Geometry: final body of the model. Coordinates: model frame, mm. A direction names the side the tool comes from. Coordinates: 2 decimals unless noted, no trailing zeros. Order: outer loops, then holes, each group sorted by start corner. A loop starts at its lowest first (then second) coordinate and runs counter-clockwise, first axis right, second up. Notation, with made-up numbers: M -8.5,65 L 3.5,65 A33 ccw 3.5,104 Z; hole C 74,6.5 d5. An arc over 180 degrees is marked long. Use CSV: the item, a comma, the result in double quotes. Start each with the question number.
Q1. Section query C-C, the plane y = 1.5. Output: boundary loops of the cut face in (x, z), and give its area (3 significant figures).
Q2. Mould query, pull axis Y, two halves, no side actions, for faces 1 (the face through (1, -1.828, -15)), 2 (the face through (-22.1, -4.1, -0.7)), 3 (the face through (22.4, -3.128, -6.2)), 4 (the face through (18, -13.128, 4)). Classes: +Y half, -Y half, draft (parallel to the pull), parting line (faces both ways), or undercut.
Q3. Section query B-B, the plane z = 30.5. Output: boundary loops of the cut face in (x, y), and give its area (3 significant figures).
Q4. Ray query, probe 1 along X at (y, z) = (-2.5, -1); probe 2 along Y at (x, z) = (-21, -10); probe 3 along Z at (x, y) = (11.5, -9.25). Return the intervals inside material, ascending.
Q5. First-contact query: P1, Ø1.5, axis at y = -11, z = 16.5, coming from the -X side; P2, Ø11.5, axis at x = -25.02, z = 0, coming from the -Y side; P3, Ø2, axis at x = -6.5, z = -4, coming from the +Y side; P4, Ø5.5, axis at x = 7.48, z = 32.5, coming from the -Y side. Flat tips, straight axial feed; report the tip coordinate or a pass-through.
Q6. Access query for faces 5 (the face through (-1, -17.128, -9)), 6 (the face through (3.51, -0.09, -29.46)), 7 (the face through (26, -5.128, -8)). Directions: +Z, -Z, +X, -X, +Y, -Y. A direction counts if a zero-diameter tool reaches every point of the face in a straight line with its end or side. Return the directions, or none.
Q7. Section query A-A, the plane z = 0. State how many separate pieces and enclosed holes the cut face has, and give its area (3 significant figures).
from build123d import *

# Parameters (mm, degrees)
F3_D            = 6
F3_COPIES_COUNT = 4
F4_R            = 5
F4_R_2          = 3
F5_DEPTH        = 6
F5_COPIES_COUNT = 4


# Not quite as in the source:
# - a pattern or mirror of a feature is missing from the dataset's text; its kind, count and spacing are read off the source's solid


with BuildPart() as f1:
    # F0 (on Top) → F1 (revolve)
    with BuildSketch(Plane.XY):
        Polygon((47.481939, -5.127659), (47.481939, 2.872341), (23.481939, 2.872341), (23.481939, -1.827659), (24.331939, -1.827659), (24.331939, -3.127659), (23.481939, -3.127659), (23.481939, -13.127659), (18.481939, -13.127659), (18.481939, -17.127659), (27.481939, -17.127659), (27.481939, -5.127659), align=None)
    revolve(axis=Axis((7.481939, -6.8666535, 0), (0, -1, 0)))

    # F3 (through all)
    with Locations(Plane(origin=(0, 2.872341, 0), x_dir=(-1, 0, 0), z_dir=(0, 1, 0))):
        with Locations((-7.481939, 32.5)):
            f3 = Hole(F3_D / 2)

    # F3_copies: F3 ×4 about axis
    f3_copies_axis = Axis((7.481939, 0, 0), (0, 1, 0))
    for i in range(1, F3_COPIES_COUNT):
        add(f3.rotate(f3_copies_axis, i * 360 / F3_COPIES_COUNT), mode=Mode.SUBTRACT)

    # F4 (on face) → F5 (cut)
    with BuildSketch(Plane(origin=(0, 2.872341, 0), x_dir=(-1, 0, 0), z_dir=(0, 1, 0))):
        with Locations((-7.481939, 32.5)):
            Circle(F4_R)
        with Locations((-7.481939, 32.5)):
            Circle(F4_R_2, mode=Mode.SUBTRACT)
    f5 = extrude(amount=-F5_DEPTH, mode=Mode.SUBTRACT)

    # F5_copies: F5 ×4 about axis
    f5_copies_axis = Axis((7.481939, 0, 0), (0, 1, 0))
    for i in range(1, F5_COPIES_COUNT):
        add(f5.rotate(f5_copies_axis, i * 360 / F5_COPIES_COUNT), mode=Mode.SUBTRACT)


solid = f1.part
Responses:
1,outline,"C 7.48,0 d80; hole C -25.02,0 d10; hole C 7.48,0 d32; hole C 7.48,-32.5 d10; hole C 7.48,32.5 d10; hole C 39.98,0 d10"
1,area,"3,910 mm²"
2,face 1,"undercut"
2,face 2,"draft"
2,face 3,"undercut"
2,face 4,"+Y half"
3,outline,"M -18.4,-5.13 L 5.25,-5.13 L 5.25,-3.13 L 2.9,-3.13 L 2.9,2.87 L -18.4,2.87 Z; M 9.72,-5.13 L 33.36,-5.13 L 33.36,2.87 L 12.06,2.87 L 12.06,-3.13 L 9.72,-3.13 Z"
3,area,"350 mm²"
4,probe 1,"x = -32.51 to -29.92, -20.12 to -9.34, 24.3 to 35.08, 44.88 to 47.47"
4,probe 2,"y = -5.13 to 2.87"
4,probe 3,"z = -19.59 to -15.49, 15.49 to 19.59"
5,P1,"stops at x = -4.84"
5,P2,"stops at y = -5.13"
5,P3,"stops at y = -13.13"
5,P4,"passes through"
6,face 5,"+Z, -Z, +X, -X, -Y"
6,face 6,"+Y"
6,face 7,"-Y"
7,separate pieces,"4"
7,enclosed holes,"0"
7,area,"374 mm²"
